Here's how the part is built. I have some questions about the finished solid (model axes, mm). Give positions to 0.01 mm unless a question says otherwise; leave off trailing zeros. Loops run counter-clockwise (first coordinate to the right, second up) from the corner with the lowest first, then second, coordinate; pieces in that order, holes last. Notation, with made-up numbers: (26.5, 9) -> (40.5, 9) arc R32 cw to (40.5, 38) -> close; hole circle Ø4 at (61.25, -30). An arc over 180 degrees is marked (long way). Answer in a Markdown table with one row per item. Add a question column.
Item 1: If I drill on line 1 (Z direction, x = -9.5, y = 0.4); line 2 (X direction, y = -1.35, z = 116); line 3 (Z direction, x = 50, y = -0.9), over which ranges is the centre line in solid material (lowest first)?
Item 2: If we section it at C-C (x = 45): Write out the boundary of the cut face in (y, z), then the cut area to 3 significant figures.
Item 3: For P1, Ø1.5, axis at x = -54, y = 0.5, coming from the -Z side; P2, Ø1.5, axis at y = 1, z = -43, coming from the -X side; P3, Ø2.5, axis at x = 8, y = 0.5, coming from the +Z side, each with a flat end and sliding along its axis, tell me the tip position at first contact or that it passes through.
Item 4: If we section it at B-B (y = 0.15): Give the number of separate pieces and of enclosed holes in the cut face, then the cut area to 3 significant figures.
Item 5: If we section it at A-A (x = 9): Write out the boundary of the cut face in (y, z), then the cut area to 3 significant figures.
Item 6: If we section it at D-D (z = -3): Write out the boundary of the cut face in (x, y), then the cut area to 3 significant figures.
```python
from build123d import *

# Parameters (mm, degrees)
SKETCH1_W           = 4.953
SKETCH1_H           = 7.62
BOSS_EXTRUDE1_DEPTH = 2.4765


with BuildPart() as part:
    # Sketch1 → Boss-Extrude1 (new, symmetric)
    with BuildSketch(Plane(origin=(0, 0, 0), x_dir=(1, 0, 0), z_dir=(0, 1, 0))):
        with BuildLine():
            Line((-49.53, 45.72), (-11.7983, 45.72))
            Line((-11.7983, 45.72), (-11.7983, 38.1))
            Line((-11.7983, 38.1), (-6.8453, 38.1))
            Line((-6.8453, 38.1), (-6.8453, 45.72))
            Line((-6.8453, 45.72), (6.8453, 45.72))
            Line((6.8453, 45.72), (6.8453, 38.1))
            Line((6.8453, 38.1), (11.7983, 38.1))
            Line((11.7983, 38.1), (11.7983, 45.72))
            Line((11.7983, 45.72), (49.53, 45.72))
            Line((49.53, 45.72), (49.53, 38.1))
            Line((49.53, 38.1), (55.626, 38.1))
            Line((55.626, 38.1), (55.626, 27.94))
            Line((55.626, 27.94), (49.53, 27.94))
            Line((49.53, 27.94), (49.53, 1.208143374))
            Line((49.53, 1.208143374), (55.626, 1.208143374))
            Line((55.626, 1.208143374), (55.626, -8.951856626))
            Line((55.626, -8.951856626), (49.53, -8.951856626))
            Line((49.53, -8.951856626), (49.53, -16.571856626))
            Line((49.53, -16.571856626), (55.626, -16.571856626))
            Line((55.626, -16.571856626), (55.626, -29.271856626))
            Line((55.626, -29.271856626), (21.019827136, -42.136821893))
            ThreePointArc((21.019827136, -42.136821893), (17.95098831, -44.911778638), (17.631953735, -49.036869377))
            Line((17.631953735, -49.036869377), (25.187729856, -73.287029113))
            ThreePointArc((25.187729856, -73.287029113), (26.234780075, -75.207903536), (27.939063878, -76.579577488))
            ThreePointArc((27.939063878, -76.579577488), (41.468907088, -82.632484358), (55.626, -87.022365809))
            Line((55.626, -87.022365809), (55.626, -132.617292876))
            Line((55.626, -132.617292876), (11.7983, -132.617292876))
            Line((11.7983, -132.617292876), (11.7983, -122.457292876))
            Line((11.7983, -122.457292876), (6.9723, -122.457292876))
            Line((6.9723, -122.457292876), (6.9723, -94.642365809))
            Line((6.9723, -94.642365809), (11.7983, -94.642365809))
            Line((11.7983, -94.642365809), (11.7983, -87.022365809))
            Line((11.7983, -87.022365809), (6.9723, -87.022365809))
            Line((6.9723, -87.022365809), (6.9723, -80.672365809))
            Line((6.9723, -80.672365809), (-6.9723, -80.672365809))
            Line((-6.9723, -80.672365809), (-6.9723, -87.022365809))
            Line((-6.9723, -87.022365809), (-11.7983, -87.022365809))
            Line((-11.7983, -87.022365809), (-11.7983, -94.642365809))
            Line((-11.7983, -94.642365809), (-6.9723, -94.642365809))
            Line((-6.9723, -94.642365809), (-6.9723, -122.457292876))
            Line((-6.9723, -122.457292876), (-11.7983, -122.457292876))
            Line((-11.7983, -122.457292876), (-11.7983, -132.617292876))
            Line((-11.7983, -132.617292876), (-49.53, -132.617292876))
            Line((-49.53, -132.617292876), (-49.53, -124.997292876))
            Line((-49.53, -124.997292876), (-55.626, -124.997292876))
            Line((-55.626, -124.997292876), (-55.626, -116.107292876))
            Line((-55.626, -116.107292876), (-49.53, -116.107292876))
            Line((-49.53, -116.107292876), (-49.53, -105.947292876))
            Line((-49.53, -105.947292876), (-55.626, -105.947292876))
            Line((-55.626, -105.947292876), (-55.626, -97.057292876))
            Line((-55.626, -97.057292876), (-49.53, -97.057292876))
            Line((-49.53, -97.057292876), (-49.53, -85.359826344))
            ThreePointArc((-49.53, -85.359826344), (-38.527111219, -81.479756652), (-27.939063878, -76.579577488))
            ThreePointArc((-27.939063878, -76.579577488), (-26.234780075, -75.207903536), (-25.187729856, -73.287029113))
            Line((-25.187729856, -73.287029113), (-17.631953735, -49.036869377))
            ThreePointArc((-17.631953735, -49.036869377), (-17.95098831, -44.911778638), (-21.019827136, -42.136821893))
            Line((-21.019827136, -42.136821893), (-55.626, -29.271856626))
            Line((-55.626, -29.271856626), (-55.626, -16.571856626))
            Line((-55.626, -16.571856626), (-49.53, -16.571856626))
            Line((-49.53, -16.571856626), (-49.53, -8.951856626))
            Line((-49.53, -8.951856626), (-55.626, -8.951856626))
            Line((-55.626, -8.951856626), (-55.626, 1.208143374))
            Line((-55.626, 1.208143374), (-49.53, 1.208143374))
            Line((-49.53, 1.208143374), (-49.53, 27.94))
            Line((-49.53, 27.94), (-55.626, 27.94))
            Line((-55.626, 27.94), (-55.626, 38.1))
            Line((-55.626, 38.1), (-49.53, 38.1))
            Line((-49.53, 38.1), (-49.53, 45.72))
        make_face()
        with Locations((9.3218, -25.461856626)):
            Rectangle(SKETCH1_W, SKETCH1_H, mode=Mode.SUBTRACT)
        with Locations((-9.3218, -25.461856626)):
            Rectangle(SKETCH1_W, SKETCH1_H, mode=Mode.SUBTRACT)
    extrude(amount=BOSS_EXTRUDE1_DEPTH, both=True)


solid = part.part
```
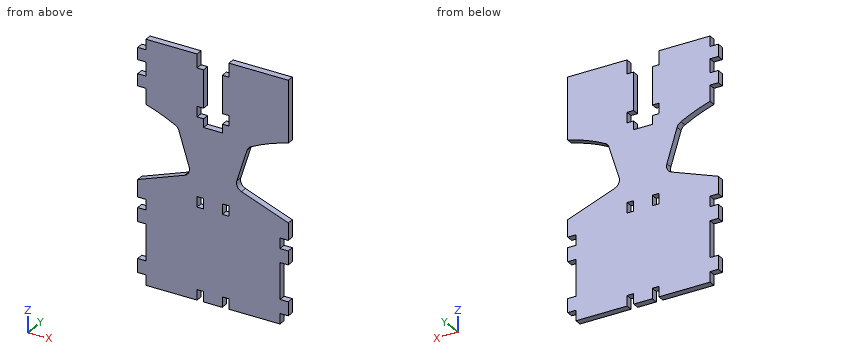
Recorded:
| question | item | result |
|---|---|---|
| 1 | line 1 | z = -38.1 to 21.65, 29.27 to 87.02, 94.64 to 122.46 |
| 1 | line 2 | x = -49.53 to -6.97, 6.97 to 55.63 |
| 1 | line 3 | z = -38.1 to -27.94, -1.21 to 8.95, 16.57 to 31.36, 85.5 to 132.62 |
| 2 | outline | (-2.48, -45.72) -> (2.48, -45.72) -> (2.48, 33.22) -> (-2.48, 33.22) -> close; (-2.48, 83.9) -> (2.48, 83.9) -> (2.48, 132.62) -> (-2.48, 132.62) -> close |
| 2 | area | 632 mm^2 |
| 3 | P1 | stops at z = -38.1 |
| 3 | P2 | stops at x = -49.53 |
| 3 | P3 | stops at z = 122.46 |
| 4 | separate pieces | 1 |
| 4 | enclosed holes | 2 |
| 4 | area | 15,000 mm^2 |
| 5 | outline | (-2.48, -38.1) -> (2.48, -38.1) -> (2.48, 21.65) -> (-2.48, 21.65) -> close; (-2.48, 29.27) -> (2.48, 29.27) -> (2.48, 87.02) -> (-2.48, 87.02) -> close; (-2.48, 94.64) -> (2.48, 94.64) -> (2.48, 122.46) -> (-2.48, 122.46) -> close |
| 5 | area | 720 mm^2 |
| 6 | outline | (-49.53, -2.48) -> (49.53, -2.48) -> (49.53, 2.48) -> (-49.53, 2.48) -> close |
| 6 | area | 491 mm^2 |
